```python
from build123d import *

# Parameters (mm, degrees)
SKETCH1_R           = 1.2
SKETCH1_R_2         = 1.225
SKETCH1_R_3         = 1.25
SKETCH1_R_4         = 1.275
SKETCH1_R_5         = 1.3
SKETCH1_R_6         = 1.6
SKETCH1_R_7         = 1.625
SKETCH1_R_8         = 1.65
SKETCH1_R_9         = 1.675
SKETCH1_R_10        = 1.7
BOSS_EXTRUDE1_DEPTH = 8
FILLET1_R           = 1


with BuildPart() as part:
    # Sketch1 → Boss-Extrude1 (new body)
    with BuildSketch(Plane(origin=(0, 0, 0), x_dir=(1, 0, 0), z_dir=(0, 1, 0))):
        Polygon((0, 0), (27, 0), (27, 4.5), (31, 4.5), (31, 11.5), (0, 11.5), align=None)
        with Locations(Location((3.5, 3.5, 0), (0, 0, 270))):
            Circle(SKETCH1_R, mode=Mode.SUBTRACT)
        with Locations(Location((8.5, 3.5, 0), (0, 0, 270))):
            Circle(SKETCH1_R_2, mode=Mode.SUBTRACT)
        with Locations(Location((13.5, 3.5, 0), (0, 0, 270))):
            Circle(SKETCH1_R_3, mode=Mode.SUBTRACT)
        with Locations(Location((18.5, 3.5, 0), (0, 0, 270))):
            Circle(SKETCH1_R_4, mode=Mode.SUBTRACT)
        with Locations(Location((23.5, 3.5, 0), (0, 0, 270))):
            Circle(SKETCH1_R_5, mode=Mode.SUBTRACT)
        with Locations(Location((3.5, 8, 0), (0, 0, 270))):
            Circle(SKETCH1_R_6, mode=Mode.SUBTRACT)
        with Locations(Location((9.5, 8, 0), (0, 0, 270))):
            Circle(SKETCH1_R_7, mode=Mode.SUBTRACT)
        with Locations(Location((15.5, 8, 0), (0, 0, 270))):
            Circle(SKETCH1_R_8, mode=Mode.SUBTRACT)
        with Locations(Location((21.5, 8, 0), (0, 0, 270))):
            Circle(SKETCH1_R_9, mode=Mode.SUBTRACT)
        with Locations(Location((27.5, 8, 0), (0, 0, 270))):
            Circle(SKETCH1_R_10, mode=Mode.SUBTRACT)
    extrude(amount=BOSS_EXTRUDE1_DEPTH)

    # Fillet1
    fillet1_edges = [part.edges().sort_by_distance(p)[0] for p in [
        (0, 4, -11.5),
        (31, 4, -11.5),
        (31, 4, -4.5),
        (27, 4, -4.5),
        (27, 4, 0),
        (0, 4, 0),
    ]]
    fillet(fillet1_edges, radius=FILLET1_R)


solid = part.part
```
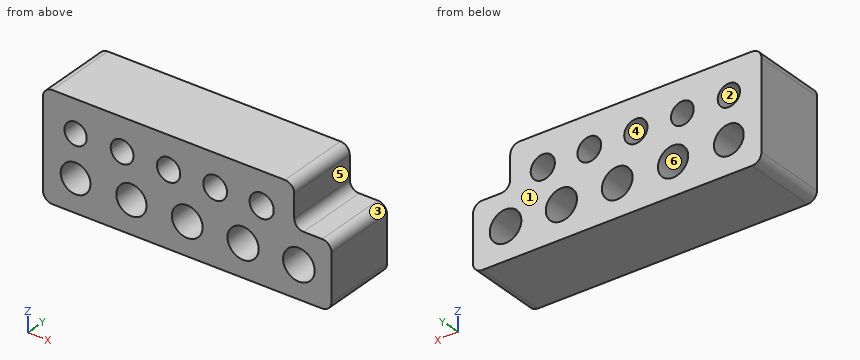
Model file for the job. Use its own axes, mm. Face numbers are marked on the shaded views. A direction names the side the tool comes from. Coordinates: 2 decimals unless noted, no trailing zeros. Order: outer loops, then holes, each group sorted by start corner. A loop starts at its lowest first (then second) coordinate and runs counter-clockwise, first axis right, second up. Notation, with made-up numbers: (41.5, -23) -> (98.5, -23) arc R27 cw to (98.5, 14) -> close; hole circle Ø3 at (-14.75, 52). An arc over 180 degrees is marked (long way). Answer as a JSON object with one key per item and string values. Group by question number.
1) Flat gauge pins, fed straight in: pin 1 (3.5 mm diameter, centred on x = 9.5, z = -8, fed in from +Y); pin 2 (0.8 mm diameter, centred on y = 5, z = -2.5, fed in from +X); pin 3 (2 mm diameter, centred on x = 29, y = 5, fed in from +Z). Where does each tip first touch, or does it go through?
2) Drill centre lines: L1, parallel to X at y = 5.5, z = -3.5 (3 decimals); L2, parallel to X at y = 4.5, z = -8 (3 decimals); L3, parallel to Z at x = 24, y = 6.75. Where is each one in solid material? Low to high.
3) Cut at B-B, the plane z = -8. Write the cut outline in (x, y) (3 decimals), then the cut area to 3 significant figures.
4) Cut at A-A, the plane x = 13.5. Write the cut outline in (y, z).
5) Which spindle directions (+Z, -Z, +X, -X, +Y, -Y) get a long thin tool onto all of the face, cutting with end or side? Do the marked faces 5 and 6. Say none if no direction does.
6) Cut at D-D, the plane x = 24. Write the cut outline in (y, z), then the cut area to 3 significant figures.
7) Cut at C-C, the plane y = 3.5. Count the separate pieces of the cut face and the enclosed holes in it, then the cut area to 3 significant figures.
8) Pull direction X, two halves, no side cores. Call the marked faces 1, 2, 3 and 4: +X half, -X half, draft (parallel to the pull), parting line (faces both ways), or undercut.
Check values:
{
 "1": {"pin 1": "stops at y = 8", "pin 2": "stops at x = 27", "pin 3": "stops at z = -4.5"},
 "2": {"L1": "x = 0 to 2.3, 4.7 to 7.275, 9.725 to 12.25, 14.75 to 17.225, 19.775 to 22.2, 24.8 to 27", "L2": "x = 0 to 1.9, 5.1 to 7.875, 11.125 to 13.85, 17.15 to 19.825, 23.175 to 25.8, 29.2 to 31", "L3": "z = -11.5 to -4.7, -2.3 to 0"},
 "3": {"outline": "(0, 0) -> (1.9, 0) -> (1.9, 8) -> (0, 8) -> close; (5.1, 0) -> (7.875, 0) -> (7.875, 8) -> (5.1, 8) -> close; (11.125, 0) -> (13.85, 0) -> (13.85, 8) -> (11.125, 8) -> close; (17.15, 0) -> (19.825, 0) -> (19.825, 8) -> (17.15, 8) -> close; (23.175, 0) -> (25.8, 0) -> (25.8, 8) -> (23.175, 8) -> close; (29.2, 0) -> (31, 0) -> (31, 8) -> (29.2, 8) -> close", "area": "116 mm²"},
 "4": {"outline": "(0, -11.5) -> (8, -11.5) -> (8, -4.75) -> (0, -4.75) -> close; (0, -2.25) -> (8, -2.25) -> (8, 0) -> (0, 0) -> close"},
 "5": {"face 5": "+Z, +X, +Y, -Y", "face 6": "+Y, -Y"},
 "6": {"outline": "(0, -11.5) -> (8, -11.5) -> (8, -4.7) -> (0, -4.7) -> close; (0, -2.3) -> (8, -2.3) -> (8, 0) -> (0, 0) -> close", "area": "72.8 mm²"},
 "7": {"separate pieces": "1", "enclosed holes": "10", "area": "270 mm²"},
 "8": {"face 1": "draft", "face 2": "undercut", "face 3": "+X half", "face 4": "undercut"}
}
